```python
from build123d import *

# Parameters (mm, degrees)
SKETCH1_R               = 12.7
SKETCH1_R_2             = 3.15
BOSS_EXTRUDE1_DEPTH     = 19.05
BOSS_EXTRUDE2_START     = -19.05
BOSS_EXTRUDE2_DEPTH     = 19.05
CUT_EXTRUDE1_REACH      = 46.45
CUT_EXTRUDE1_END_RADIUS = 3.15
SKETCH3_R               = 1.55


with BuildPart() as part:
    # Sketch1 → Boss-Extrude1 (new body)
    with BuildSketch(Plane(origin=(0, 0, 0), x_dir=(0, 0, -1), z_dir=(1, 0, 0))):
        with Locations(Location((0, 0, 0), (0, 0, 180))):
            Circle(SKETCH1_R)
        with Locations(Location((0, 0, 0), (0, 0, 180))):
            Circle(SKETCH1_R_2, mode=Mode.SUBTRACT)
    extrude(amount=BOSS_EXTRUDE1_DEPTH)

    # Sketch2 → Boss-Extrude2 (add)
    with BuildSketch(Plane(origin=(19.05, 0, 0), x_dir=(0, 0, -1), z_dir=(1, 0, 0)).offset(BOSS_EXTRUDE2_START)):
        with BuildLine():
            Line((12.7, -25.4), (12.7, 0))
            ThreePointArc((12.7, 0), (0, -12.7), (-12.7, 0))
            Line((-12.7, 0), (-12.7, -25.4))
            Line((-12.7, -25.4), (12.7, -25.4))
        make_face()
    extrude(amount=BOSS_EXTRUDE2_DEPTH)

    # Cut-Extrude1: up to this cylinder (the profile starts outside it)
    cut_extrude1_end = Plane(origin=(9.525, 0, 0), z_dir=(-1, 0, 0)) * Cylinder(CUT_EXTRUDE1_END_RADIUS, 100.2, mode=Mode.PRIVATE)
    # Sketch3 → Cut-Extrude1 (cut, up to the surface)
    with BuildSketch(Plane(origin=(0, 12.7, 0), x_dir=(1, 0, 0), z_dir=(0, 1, 0)), mode=Mode.PRIVATE) as cut_extrude1_sk1:
        with Locations(Location((9.525, 0, 0), (0, 0, 270))):
            Circle(SKETCH3_R)
    cut_extrude1_tool1 = extrude(cut_extrude1_sk1.sketch, amount=-CUT_EXTRUDE1_REACH, mode=Mode.PRIVATE) - cut_extrude1_end
    add(cut_extrude1_tool1.solids().sort_by_distance((9.525, 12.7, 0))[0], mode=Mode.SUBTRACT)


solid = part.part
```
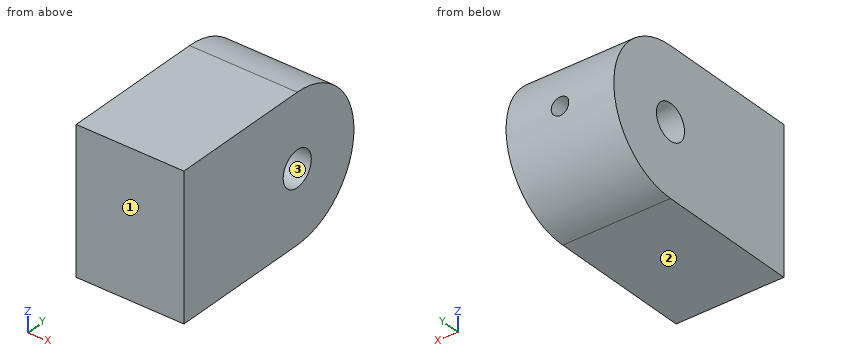
Model file for the job. Use its own axes, mm. Face numbers are marked on the shaded views. Coordinates: 2 decimals unless noted, no trailing zeros. Loops run counter-clockwise (first coordinate to the right, second up) from the corner with the lowest first, then second, coordinate; pieces in that order, holes last. Notation, with made-up numbers: (19.25, -16) -> (23.25, -16) arc R21 cw to (23.25, 6) -> close; hole circle Ø10 at (-37.75, 37). An arc over 180 degrees is marked (long way). Answer as a JSON object with one key per item and string values.
Q1. Pull direction Y, two halves, no side cores. Call the marked faces 1, 2 and 3: released by +Y, released by -Y, zero draft, split by the parting line, or undercut.
Report:
{"face 1": "released by -Y", "face 2": "zero draft", "face 3": "undercut"}
Q2. Cut at A-A (z = 0). List the corners of the cut face in (x, y) (3 decimals).
Report:
{"outline": "(0, -25.4) -> (19.05, -25.4) -> (19.05, -3.15) -> (0, -3.15) -> close; (0, 3.15) -> (7.975, 3.15) -> (7.975, 12.7) -> (0, 12.7) -> close; (11.075, 3.15) -> (19.05, 3.15) -> (19.05, 12.7) -> (11.075, 12.7) -> close"}
Q3. Probe probe 1 along Y at (x, z) = (13.25, 0); probe 2 along Y at (x, z) = (13.75, 2.5); probe 3 along Y at (x, z) = (7.5, 5). List the from-to ranges inside material, lowest first.
Report:
{"probe 1": "y = -25.4 to -3.15, 3.15 to 12.7", "probe 2": "y = -25.4 to -1.92, 1.92 to 12.45", "probe 3": "y = -25.4 to 11.67"}
Q4. Cut at C-C (z = -2.75). List the corners of the cut face in (x, y).
Report:
{"outline": "(0, -25.4) -> (19.05, -25.4) -> (19.05, -1.54) -> (0, -1.54) -> close; (0, 1.54) -> (19.05, 1.54) -> (19.05, 12.4) -> (0, 12.4) -> close"}
Q5. Cut at B-B (x = 6.5). List the corners of the cut face in (y, z).
Report:
{"outline": "(-25.4, -12.7) -> (0, -12.7) arc R12.7 ccw to (0, 12.7) -> (-25.4, 12.7) -> close; hole circle Ø6.3 at (0, 0)"}
Q6. Cut at D-D (z = -8.25). List the corners of the cut face in (x, y).
Report:
{"outline": "(0, -25.4) -> (19.05, -25.4) -> (19.05, 9.66) -> (0, 9.66) -> close"}
Q7. Flat gauge pins, fed straight in: P1, Ø3, axis at x = 6, z = -9, coming from the +Y side; P2, Ø2.5, axis at x = 9.525, z = 0, coming from the +Y side; P3, Ø6, axis at y = 0, z = 10, coming from the -X side. Where does each tip first touch, or does it go through?
Report:
{"P1": "stops at y = 10.25", "P2": "stops at y = -2.89", "P3": "stops at x = 0"}
